from build123d import *

# Parameters (mm, degrees)
BASE_EXTRUDE_DEPTH      = 20
FILLET1_R               = 10
FILLET2_R               = 10
CUT_EXTRUDE1_DEPTH      = 181.430735794
CUT_EXTRUDE1_DEPTH_BACK = 181.430735794
SKETCH4_R               = 6.25


with BuildPart() as part:
    # Sketch1 → Base-Extrude (new body)
    with BuildSketch(Plane.XY):
        Polygon((145.351370521, 25), (5.351370521, 37.5), (-24.64607099, 37.5), (-24.64607099, 10), (0.35392901, 10), (0.35392901, -10), (-24.64607099, -10), (-24.64607099, -37.5), (0.35392901, -37.5), (140.35392901, -25), (175.35392901, -25), (175.35392901, -10), (140.35392901, -10), (140.35392901, 10), (175.35392901, 10), (175.35392901, 25), align=None)
        Polygon((120.35392901, 11.726043432), (20.35392901, 20.65461486), (20.35392901, -20.65461486), (120.35392901, -11.726043432), align=None, mode=Mode.SUBTRACT)
    extrude(amount=BASE_EXTRUDE_DEPTH)

    # Fillet1
    # the kernel refuses this fillet: 10 mm, written as the material it takes off along each edge
    with BuildSketch(Plane(origin=(175.35392901, -15, 0), x_dir=(0, 0, 1), z_dir=(0, 1, 0)), Plane(origin=(175.35392901, -50, 0), x_dir=(0, 0, 1), z_dir=(0, 1, 0))) as fillet1_piece_1:
        with BuildLine():
            CenterArc((FILLET1_R, -FILLET1_R), FILLET1_R, 90, 90)
            Line((0, -FILLET1_R), (0, 0))
            Line((0, 0), (FILLET1_R, 0))
        make_face()
    extrude(amount=65, mode=Mode.SUBTRACT)
    with BuildSketch(Plane(origin=(-24.64607099, 15, 0), x_dir=(0, 0, 1), z_dir=(0, -1, 0)), Plane(origin=(-24.64607099, 62.5, 0), x_dir=(0, 0, 1), z_dir=(0, -1, 0))) as fillet1_piece_2:
        with BuildLine():
            CenterArc((FILLET1_R, -FILLET1_R), FILLET1_R, 90, 90)
            Line((0, -FILLET1_R), (0, 0))
            Line((0, 0), (FILLET1_R, 0))
        make_face()
    extrude(amount=77.5, mode=Mode.SUBTRACT)
    with BuildSketch(Plane(origin=(-24.64607099, 15, 20), x_dir=(0, 0, -1), z_dir=(0, -1, 0)), Plane(origin=(-24.64607099, 62.5, 20), x_dir=(0, 0, -1), z_dir=(0, -1, 0))) as fillet1_piece_3:
        with BuildLine():
            CenterArc((FILLET1_R, FILLET1_R), FILLET1_R, 180, 90)
            Line((0, FILLET1_R), (0, 0))
            Line((0, 0), (FILLET1_R, 0))
        make_face()
    extrude(amount=77.5, mode=Mode.SUBTRACT)
    with BuildSketch(Plane(origin=(175.35392901, -50, 20), x_dir=(0, 0, -1), z_dir=(0, 1, 0)), Plane(origin=(175.35392901, -15, 20), x_dir=(0, 0, -1), z_dir=(0, 1, 0))) as fillet1_piece_4:
        with BuildLine():
            CenterArc((FILLET1_R, FILLET1_R), FILLET1_R, 180, 90)
            Line((0, FILLET1_R), (0, 0))
            Line((0, 0), (FILLET1_R, 0))
        make_face()
    extrude(amount=65, mode=Mode.SUBTRACT)

    # Fillet2
    fillet2_edges = [part.edges().sort_by_distance(p)[0] for p in [
        (120.35392901, -11.726043432, 10),
        (120.35392901, 11.726043432, 10),
        (20.35392901, 20.65461486, 10),
        (20.35392901, -20.65461486, 10),
    ]]
    fillet(fillet2_edges, radius=FILLET2_R)

    # Sketch4 → Cut-Extrude1 (cut, two sides: drawn at the far end of the back side and taken through both)
    with BuildSketch(Plane(origin=(0, 0, 0), x_dir=(1, 0, 0), z_dir=(0, 1, 0)).offset(-CUT_EXTRUDE1_DEPTH_BACK)):
        with Locations((165.35392901, -10)):
            Circle(SKETCH4_R)
        with Locations(Location((-14.64607099, -10, 0), (0, 0, 270))):
            Circle(SKETCH4_R)
    extrude(amount=CUT_EXTRUDE1_DEPTH + CUT_EXTRUDE1_DEPTH_BACK, mode=Mode.SUBTRACT)


solid = part.part
Source: CAD feature listing. Evaluate the final solid. Frame: model axes, mm. A direction names the side the tool comes from. Coordinates: 2 decimals unless noted, no trailing zeros. Loops run counter-clockwise (first coordinate to the right, second up) from the corner with the lowest first, then second, coordinate; pieces in that order, holes last. Notation, with made-up numbers: (52, 60.5) - (57, 60.5) arc R34 ccw to (57, 91.5) - close; hole circle Ø6 at (5, 67.25). An arc over 180 degrees is marked (long way). One line per question, with ' | ' between items.
1) Set-up query: faces 4 (the face through (154, -10, 10)), 5 (the face through (154, -25, 10)), 6 (the face through (20.354, 0, 10)). Return all of +Z, -Z, +X, -X, +Y, -Y with unobstructed straight access to the full face (end or side cutting, diameter ignored); none if empty.
Report:
face 4: +Z, -Z, +X | face 5: +Z, -Z, +X, -Y | face 6: +Z, -Z
2) Pull-direction query (Z, two-part tool) for faces 1 (the face through (175.35, 17.39, 10.22)), 2 (the face through (-7, -37.5, 10)), 3 (the face through (171.315, -17.605, 8.123)); classes: released by +Z, released by -Z, zero draft, split by the parting line, or undercut.
Report:
face 1: split by the parting line | face 2: zero draft | face 3: undercut
3) Line query: line 1 along Y through (x, z) = (148, 3.5); line 2 along Y through (x, z) = (-1.5, 15.75); line 3 along X through (y, z) = (20, 14). Output: solid intervals per line, ascending.
Report:
line 1: y = -25 to -10, 10 to 25 | line 2: y = -37.5 to -10, 10 to 37.5 | line 3: x = -23.81 to -19.45, -9.84 to 160.55, 170.16 to 174.52
4) Section B-B, the plane x = 52.5. Return loops of the section in (y, z), then the cut area to 3 significant figures.
Report:
outline: (-32.84, 0) - (-17.78, 0) - (-17.78, 20) - (-32.84, 20) - close; (17.78, 0) - (33.29, 0) - (33.29, 20) - (17.78, 20) - close | area: 611 mm²
5) Section D-D, the plane x = 161.5. Return loops of the section in (y, z), then the cut area to 3 significant figures.
Report:
outline: (-25, 0) - (-10, 0) - (-10, 5.08) - (-25, 5.08) - close; (-25, 14.92) - (-10, 14.92) - (-10, 20) - (-25, 20) - close; (10, 0) - (25, 0) - (25, 5.08) - (10, 5.08) - close; (10, 14.92) - (25, 14.92) - (25, 20) - (10, 20) - close | area: 305 mm²
6) Section A-A, the plane y = -0.5. Return loops of the section in (x, z).
Report:
outline: (0.35, 0) - (20.35, 0) - (20.35, 20) - (0.35, 20) - close; (120.35, 0) - (140.35, 0) - (140.35, 20) - (120.35, 20) - close
7) Section C-C, the plane z = 18. Return loops of the section in (x, y), then the cut area to 3 significant figures.
Report:
outline: (-20.65, -37.5) - (0.35, -37.5) - (140.35, -25) - (171.35, -25) - (171.35, -10) - (140.35, -10) - (140.35, 10) - (171.35, 10) - (171.35, 25) - (145.35, 25) - (5.35, 37.5) - (-20.65, 37.5) - (-20.65, 10) - (0.35, 10) - (0.35, -10) - (-20.65, -10) - close; hole (20.35, -9.72) arc R10 ccw to (31.24, -19.68) - (111.24, -12.54) arc R10 ccw to (120.35, -2.58) - (120.35, 2.58) arc R10 ccw to (111.24, 12.54) - (31.24, 19.68) arc R10 ccw to (20.35, 9.72) - close | area: 7,750 mm²
8) First-contact query: P1, Ø10, axis at y = 3.5, z = 13.5, coming from the -X side; P2, Ø1.5, axis at x = 102.5, z = 3, coming from the +Y side; P3, Ø10, axis at x = 152.5, z = 9.5, coming from the -Y side. Flat tips, straight axial feed; report the tip coordinate or a pass-through.
Report:
P1: stops at x = 0.35 | P2: stops at y = 28.89 | P3: stops at y = -25
